```python
from build123d import *

# Parameters (mm, degrees)
SKETCH1_W           = 50
SKETCH1_H           = 50
BOSS_EXTRUDE1_DEPTH = 2.5
SKETCH2_R           = 1.525
CUT_EXTRUDE1_DEPTH  = 97.5
SKETCH6_R           = 3
CUT_EXTRUDE2_DEPTH  = 97.5
SKETCH7_R           = 4.575
SKETCH7_R_2         = 3.325
BOSS_EXTRUDE2_DEPTH = 7
FILLET1_R           = 5
FILLET2_R           = 2.25
CHAMFER1_SIZE       = 0.5
FILLET3_R           = 0.25


with BuildPart() as part:
    # Sketch1 → Boss-Extrude1 (new body)
    with BuildSketch(Plane(origin=(0, 0, 0), x_dir=(1, 0, 0), z_dir=(0, 1, 0))):
        Rectangle(SKETCH1_W, SKETCH1_H)
    extrude(amount=BOSS_EXTRUDE1_DEPTH)

    # Sketch2 → Cut-Extrude1 (cut)
    with BuildSketch(Plane(origin=(0, 2.5, 0), x_dir=(1, 0, 0), z_dir=(0, 1, 0))):
        with Locations(Location((0, 0, 0), (0, 0, 270))):
            Circle(SKETCH2_R)
    extrude(amount=-CUT_EXTRUDE1_DEPTH, mode=Mode.SUBTRACT)

    # Sketch6 → Cut-Extrude2 (cut)
    with BuildSketch(Plane(origin=(0, 2.5, 0), x_dir=(1, 0, 0), z_dir=(0, 1, 0))):
        with Locations(Location((-18.98959236, 18.98959236, 0), (0, 0, 270))):
            Circle(SKETCH6_R)
        with Locations(Location((18.98959236, 18.98959236, 0), (0, 0, 270))):
            Circle(SKETCH6_R)
        with Locations(Location((18.98959236, -18.98959236, 0), (0, 0, 270))):
            Circle(SKETCH6_R)
        with Locations(Location((-18.98959236, -18.98959236, 0), (0, 0, 270))):
            Circle(SKETCH6_R)
    extrude(amount=-CUT_EXTRUDE2_DEPTH, mode=Mode.SUBTRACT)

    # Sketch7 → Boss-Extrude2 (add)
    with BuildSketch(Plane(origin=(0, 2.5, 0), x_dir=(1, 0, 0), z_dir=(0, 1, 0))):
        with Locations(Location((0, 0, 0), (0, 0, 90))):
            Circle(SKETCH7_R)
        with Locations(Location((0, 0, 0), (0, 0, 270))):
            Circle(SKETCH7_R_2, mode=Mode.SUBTRACT)
    extrude(amount=BOSS_EXTRUDE2_DEPTH)

    # Fillet1
    fillet1_edges = [part.edges().sort_by_distance(p)[0] for p in [
        (0, 2.5, 4.575),
    ]]
    fillet(fillet1_edges, radius=FILLET1_R)

    # Fillet2
    fillet2_edges = [part.edges().sort_by_distance(p)[0] for p in [
        (-25, 2.5, 0),
        (0, 2.5, 25),
        (25, 2.5, 0),
        (0, 2.5, -25),
    ]]
    fillet(fillet2_edges, radius=FILLET2_R)

    # Chamfer1
    chamfer1_edges = [part.edges().sort_by_distance(p)[0] for p in [
        (-18.98959236, 2.5, 15.98959236),
        (18.98959236, 2.5, 15.98959236),
        (18.98959236, 2.5, -21.98959236),
        (-18.98959236, 2.5, -21.98959236),
    ]]
    chamfer(chamfer1_edges, length=CHAMFER1_SIZE)

    # Fillet3
    fillet3_edges = [part.edges().sort_by_distance(p)[0] for p in [
        (0, 9.5, -3.325),
    ]]
    fillet(fillet3_edges, radius=FILLET3_R)


solid = part.part
```
Model file for the job. Use its own axes, mm. A direction names the side the tool comes from. Give positions to 0.01 mm unless a question says otherwise; leave off trailing zeros. Write each loop counter-clockwise with the first axis right and the second up, starting at its lowest first coordinate (ties: lowest second). Pieces come first, ordered by that corner, then holes. Notation, with made-up numbers: (-21, 15) -> (24, 15) arc R5 cw to (24, 19) -> close; hole circle Ø2 at (6, 72). An arc over 180 degrees is marked (long way). Use CSV: the item, a comma, the result in double quotes. Start each with the question number.
1) Cut at A-A on z = 0. List the corners of the cut face in (x, y) (3 decimals), plus the area to 3 significant figures.
2) Cut at D-D on z = 13.5. List the corners of the cut face in (x, y), plus the area to 3 significant figures.
3) Drill centre lines: L1, parallel to X at y = 7.5, z = 0 (3 decimals); L2, parallel to Y at x = -13.5, z = -7; L3, parallel to X at y = 1.05, z = 0 (3 decimals). Where is each one in solid material? Low to high.
4) Two-plate mould, pull along X, no slides. Class faces 1 (the cylindrical face through (-0.93, 1.27, -1.21)), 2 (the cylindrical face through (24.32, 1.86, -0.35)), 3 (the flat face through (0, 0, 5)): released by +X, released by -X, zero draft, split by the parting line, or undercut.
5) Cut at C-C on y = 1. List the corners of the cut face in (x, z) (3 decimals).
6) Pin check, flat tips, straight feed: P1, Ø12, axis at x = -18, z = 9, coming from the +Y side; P2, Ø1, axis at y = 2, z = -19, coming from the +X side. Stop position of each tip, or through.
7) Tool access for faces 4 (the cylindrical face through (-3.246, 5.828, -0.721)), 5 (the cylindrical face through (0.35, 1.86, 24.32)): list every direction of +Z, -Z, +X, -X, +Y, -Y with a clear straight run to the whole face (end or side of a thin tool).
8) Cut at B-B on x = 0. List the corners of the cut face in (y, z) (3 decimals).
Final values:
1,outline,"(-25, 0) -> (-1.525, 0) -> (-1.525, 2.5) -> (-3.325, 2.5) -> (-3.325, 9.25) arc R0.25 ccw to (-3.575, 9.5) -> (-4.575, 9.5) -> (-4.575, 7.5) arc R5 cw to (-9.575, 2.5) -> (-22.75, 2.5) arc R2.25 ccw to (-25, 0.25) -> close; (1.525, 0) -> (25, 0) -> (25, 0.25) arc R2.25 ccw to (22.75, 2.5) -> (9.575, 2.5) arc R5 cw to (4.575, 7.5) -> (4.575, 9.5) -> (3.575, 9.5) arc R0.25 ccw to (3.325, 9.25) -> (3.325, 2.5) -> (1.525, 2.5) -> close"
1,area,"143 mm2"
2,outline,"(-25, 0) -> (25, 0) -> (25, 0.25) arc R2.25 ccw to (22.75, 2.5) -> (-22.75, 2.5) arc R2.25 ccw to (-25, 0.25) -> close"
2,area,"123 mm2"
3,L1,"x = -4.575 to -3.325, 3.325 to 4.575"
3,L2,"y = 0 to 2.5"
3,L3,"x = -24.853 to -1.525, 1.525 to 24.853"
4,face 1,"undercut"
4,face 2,"released by +X"
4,face 3,"zero draft"
5,outline,"(-24.871, -24.871) -> (24.871, -24.871) -> (24.871, 24.871) -> (-24.871, 24.871) -> close; hole circle Ø6 at (-18.99, -18.99); hole circle Ø6 at (-18.99, 18.99); hole circle Ø3.05 at (0, 0); hole circle Ø6 at (18.99, -18.99); hole circle Ø6 at (18.99, 18.99)"
6,P1,"stops at y = 2.5"
6,P2,"stops at x = 24.62"
7,face 4,"+Y"
7,face 5,"+Z, +X, -X, +Y"
8,outline,"(0, -25) -> (0.25, -25) arc R2.25 ccw to (2.5, -22.75) -> (2.5, -9.575) arc R5 cw to (7.5, -4.575) -> (9.5, -4.575) -> (9.5, -3.575) arc R0.25 ccw to (9.25, -3.325) -> (2.5, -3.325) -> (2.5, -1.525) -> (0, -1.525) -> close; (0, 1.525) -> (2.5, 1.525) -> (2.5, 3.325) -> (9.25, 3.325) arc R0.25 ccw to (9.5, 3.575) -> (9.5, 4.575) -> (7.5, 4.575) arc R5 cw to (2.5, 9.575) -> (2.5, 22.75) arc R2.25 ccw to (0.25, 25) -> (0, 25) -> close"
